Geometry: final body of the model. Coordinates: model frame, mm. A direction names the side the tool comes from. Give positions to 0.01 mm unless a question says otherwise; leave off trailing zeros. Write each loop counter-clockwise with the first axis right and the second up, starting at its lowest first coordinate (ties: lowest second). Pieces come first, ordered by that corner, then holes.
from build123d import *

# Parameters (mm, degrees)
SKETCH_R     = 4.75
SKETCH_R_2   = 2
PAD_DEPTH    = 5
SKETCH001_R  = 2.35
PAD001_DEPTH = 5
SKETCH002_R  = 3.5
POCKET_DEPTH = 3
CHAMFER_SIZE = 1.5


with BuildPart() as part:
    # Sketch → Pad (new body)
    with BuildSketch(Plane.XY):
        with BuildLine():
            ThreePointArc((-15, 34.369318), (0, -37.5), (15, 34.369318))
            Line((15, 32.5), (15, 34.369318))
            Line((-15, 32.5), (15, 32.5))
            Line((-15, 34.369318), (-15, 32.5))
        make_face()
        Circle(SKETCH_R, mode=Mode.SUBTRACT)
        with Locations((-9, 24.5)):
            Circle(SKETCH_R_2, mode=Mode.SUBTRACT)
        with Locations((9, 24.5)):
            Circle(SKETCH_R_2, mode=Mode.SUBTRACT)
        with Locations((-17.5, -8)):
            Circle(SKETCH_R_2, mode=Mode.SUBTRACT)
        with Locations((17.5, -8)):
            Circle(SKETCH_R_2, mode=Mode.SUBTRACT)
    extrude(amount=PAD_DEPTH)

    # Sketch001 (on Face11 of Pad) → Pad001 (join)
    with BuildSketch(Plane.XY.offset(5)):
        with Locations((17.320508, 10)):
            Circle(SKETCH001_R)
        with Locations((-17.320508, 10)):
            Circle(SKETCH001_R)
        with Locations((0, -20)):
            Circle(SKETCH001_R)
    extrude(amount=PAD001_DEPTH)

    # Sketch002 (on Face5 of Pad001) → Pocket (cut)
    with BuildSketch(Plane.XY.offset(5)):
        with Locations((-9, 24.5)):
            Circle(SKETCH002_R)
        with Locations((9, 24.5)):
            Circle(SKETCH002_R)
        with Locations((17.5, -8)):
            Circle(SKETCH002_R)
        with Locations((-17.5, -8)):
            Circle(SKETCH002_R)
    extrude(amount=-POCKET_DEPTH, mode=Mode.SUBTRACT)

    # Chamfer
    chamfer_edges = [part.edges().sort_by_distance(p)[0] for p in [
        (0, -37.5, 0),
    ]]
    chamfer(chamfer_edges, length=CHAMFER_SIZE)


solid = part.part
Q1. Ray query, line 1 along X through (y, z) = (-8, 0.65); line 2 along Z through (x, y) = (-17, 1); line 3 along X through (y, z) = (-8, 0.6). Return the intervals inside material, ascending.
Filled sheet:
line 1: x = -35.77 to -19.5, -15.5 to 15.5, 19.5 to 35.77
line 2: z = 0 to 5
line 3: x = -35.71 to -19.5, -15.5 to 15.5, 19.5 to 35.71
Q2. Pin query (flat end, axial travel): P1, Ø5.5, axis at x = 5.5, z = 1.5, coming from the +Y side; P2, Ø1.5, axis at y = -26, z = 7.5, coming from the +X side; P3, Ø6, axis at x = 2, z = 6, coming from the -Y side; P4, Ø2, axis at y = 33, z = 1.5, coming from the +X side. Return the tip coordinate at first contact, or that it passes through.
Filled sheet:
P1: stops at y = 32.5
P2: passes through
P3: stops at y = -37.5
P4: stops at x = 19.55
Q3. Pull-direction query (X, two-part tool) for faces 4 (the cylindrical face through (-11.58, 26.865, 3.521)), 5 (the cylindrical face through (-0.509, -22.294, 7.465)), 6 (the flat face through (0, -20, 10)); classes: released by +X, released by -X, zero draft, split by the parting line, or undercut.
Filled sheet:
face 4: undercut
face 5: split by the parting line
face 6: zero draft
Q4. Section A-A on x = 0. Output: boundary loops of the cut face in (y, z), plus the area to 3 significant figures.
Filled sheet:
outline: (-37.5, 1.5) - (-36, 0) - (-4.75, 0) - (-4.75, 5) - (-17.65, 5) - (-17.65, 10) - (-22.35, 10) - (-22.35, 5) - (-37.5, 5) - close; (4.75, 0) - (32.5, 0) - (32.5, 5) - (4.75, 5) - close
area: 325 mm2
Q5. Section B-B on z = 7.25. Output: boundary loops of the cut face in (x, y), plus the area to 3 significant figures.
Filled sheet:
outline: circle Ø4.7 at (-17.32, 10); circle Ø4.7 at (0, -20); circle Ø4.7 at (17.32, 10)
area: 52.0 mm2
Q6. Access query for faces 1 (the cylindrical face through (6.42, 26.865, 3.521)), 2 (the flat face through (-15, 33, 3)), 3 (the conical face through (-1.385, -36.213, 0.239)). Directions: +Z, -Z, +X, -X, +Y, -Y. A direction counts if a zero-diameter tool reaches every point of the face in a straight line with its end or side. Return the directions, or none.
Filled sheet:
face 1: +Z
face 2: +Z, -Z, +Y
face 3: -Z
